from build123d import *


with BuildPart() as part:
    # Sketch1 → Revolve1 (revolve)
    with BuildSketch(Plane.XY, mode=Mode.PRIVATE) as revolve1_sk:
        with BuildLine():
            Line((9.641935015, 3.175), (10.795, 3.175))
            ThreePointArc((10.795, 3.175), (11.693025612, 3.546974388), (12.065, 4.445))
            Line((12.065, 4.445), (12.065, 5.715))
            ThreePointArc((12.065, 5.715), (12.436974388, 6.613025612), (13.335, 6.985))
            Line((13.335, 6.985), (67.006445218, 6.985))
            ThreePointArc((67.006445218, 6.985), (64.752732969, 3.810778182), (63.9572, 0))
            Line((63.9572, 0), (-9.3472, 0))
            ThreePointArc((-9.3472, 0), (-2.003193278, 9.13002544), (8.488593506, 3.913301435))
            ThreePointArc((8.488593506, 3.913301435), (8.957229669, 3.375383906), (9.641935015, 3.175))
        make_face()
    revolve(revolve1_sk.sketch.rotate(Axis((-323.172189465, 0, 0), (1, 0, 0)), 90), axis=Axis((-323.172189465, 0, 0), (1, 0, 0)))


solid = part.part
Read the model definition and answer for the solid it produces. Units are mm, in the model's axes. Coordinates: 2 decimals unless noted, no trailing zeros. Loops run counter-clockwise (first coordinate to the right, second up) from the corner with the lowest first, then second, coordinate; pieces in that order, holes last. Notation, with made-up numbers: (-36.5, 22.5) - (-21.5, 22.5) arc R16 cw to (-21.5, 49.5) - close; hole circle Ø7 at (79.5, 55). An arc over 180 degrees is marked (long way). Answer in a Markdown table with one row per item.
Q1. Find section D-D on x = -0.5. Write down the section's boundary in (y, z).
Here are the results:
| item | result |
|---|---|
| outline | circle Ø18.67 at (0, 0) |
Q2. Find section A-A on y = 0. Write down the section's boundary in (x, z) (3 decimals).
Here are the results:
| item | result |
|---|---|
| outline | (8.489, -3.913) arc R1.27 cw to (9.642, -3.175) - (10.795, -3.175) arc R1.27 cw to (12.065, -4.445) - (12.065, -5.715) arc R1.27 ccw to (13.335, -6.985) - (67.006, -6.985) arc R9.525 cw to (67.006, 6.985) - (13.335, 6.985) arc R1.27 ccw to (12.065, 5.715) - (12.065, 4.445) arc R1.27 cw to (10.795, 3.175) - (9.642, 3.175) arc R1.27 cw to (8.489, 3.913) arc R9.347 ccw (long way) to start |
Q3. Given P1, Ø4, axis at y = 7.5, z = 5.5, coming from the -X side; P2, Ø1.5, axis at x = 43.5, y = 5, coming from the -Z side; P3, Ø5, axis at x = 48.5, z = 1.5, coming from the +Y side (3 decimals), each flat-ended and moving along its own axis, determine where each tip first touches the part or whether it passes through.
Here are the results:
| item | result |
|---|---|
| P1 | stops at x = -5.84 |
| P2 | stops at z = -5.54 |
| P3 | stops at y = 6.985 |
Q4. Find section C-C on x = 21. Write down the section's boundary in (y, z) (3 decimals), plus the area to 3 significant figures.
Here are the results:
| item | result |
|---|---|
| outline | circle Ø13.97 at (0, 0) |
| area | 153 mm^2 |
Q5. The mould has two halves that part along X. Classify faces 1 (the cylindrical face through (10.23, 1.93, -2.52)), 2 (the cylindrical face through (40.546, -6.926, -0.909)): pulls with the +X half, pulls with the -X half, needs draft (parallel to the pull), parting line crosses it, or undercut.
Here are the results:
| item | result |
|---|---|
| face 1 | undercut |
| face 2 | needs draft |
Q6. Straight lines are drawn through the part: line 1 along X through (y, z) = (5.25, 3.5); line 2 along X through (y, z) = (-5.25, -1) (3 decimals); line 3 along Z through (x, y) = (54, 4). For each, find the intervals that lie inside material, in ascending order. Write a range as [from, to].
Here are the results:
| item | result |
|---|---|
| line 1 | x = [-6.9, 6.9], [12.21, 66.35] |
| line 2 | x = [-7.669, 7.669], [12.065, 65.598] |
| line 3 | z = [-5.73, 5.73] |
